from build123d import *

# Parameters (mm, degrees)
BOSS_EXTRUDE1_DEPTH = 88.9
FILLET1_R           = 10.16
CUT_EXTRUDE1_REACH  = 76.71
SKETCH2_R           = 3.429
SKETCH2_R_2         = 2.54
SKETCH2_W           = 45.212
SKETCH2_H           = 26.416
CUT_EXTRUDE3_REACH  = 83.026
SKETCH4_R           = 1.27
SKETCH4_W           = 27.94
SKETCH4_H           = 25.4


with BuildPart() as part:
    # Sketch1 → Boss-Extrude1 (new body)
    with BuildSketch(Plane(origin=(0, 0, 0), x_dir=(0, 0, -1), z_dir=(1, 0, 0))):
        Polygon((0, 0), (0, 23.315129188), (30.532870812, 53.848), (74.676, 53.848), (74.676, 0), (77.851, 0), (77.851, 57.023), (29.217742751, 57.023), (-3.175, 24.630257249), (-3.175, 0), align=None)
    extrude(amount=BOSS_EXTRUDE1_DEPTH)

    # Fillet1
    fillet1_edges = [part.edges().sort_by_distance(p)[0] for p in [
        (44.45, 24.630257249, 3.175),
        (44.45, 57.023, -29.217742751),
        (44.45, 57.023, -77.851),
        (44.45, 53.848, -74.676),
        (44.45, 53.848, -30.532870812),
        (44.45, 23.315129188, 0),
    ]]
    fillet(fillet1_edges, radius=FILLET1_R)

    # Sketch2 → Cut-Extrude1 (cut, up to next)
    with BuildSketch(Plane(origin=(0, 13.902628624, 13.902628624), x_dir=(1, 0, 0), z_dir=(0, 0.707106781, 0.707106781)), mode=Mode.PRIVATE) as cut_extrude1_sk1:
        with Locations(Location((75.819, 46.966285953, 0), (0, 0, 270))):  # turned: the seam where the file's is
            Circle(SKETCH2_R)
    cut_extrude1_tool1 = extrude(cut_extrude1_sk1.sketch, amount=-CUT_EXTRUDE1_REACH, mode=Mode.PRIVATE) & part.part
    add(cut_extrude1_tool1.solids().sort_by_distance((75.819, 47.112808, -19.307551))[0], mode=Mode.SUBTRACT)
    # Sketch2 → Cut-Extrude1 (cut, up to next)
    with BuildSketch(Plane(origin=(0, 13.902628624, 13.902628624), x_dir=(1, 0, 0), z_dir=(0, 0.707106781, 0.707106781)), mode=Mode.PRIVATE) as cut_extrude1_sk2:
        with Locations(Location((75.819, 29.186285953, 0), (0, 0, 270))):  # turned: the seam where the file's is
            Circle(SKETCH2_R)
    cut_extrude1_tool2 = extrude(cut_extrude1_sk2.sketch, amount=-CUT_EXTRUDE1_REACH, mode=Mode.PRIVATE) & part.part
    add(cut_extrude1_tool2.solids().sort_by_distance((75.819, 34.540449, -6.735192))[0], mode=Mode.SUBTRACT)
    # Sketch2 → Cut-Extrude1 (cut, up to next)
    with BuildSketch(Plane(origin=(0, 13.902628624, 13.902628624), x_dir=(1, 0, 0), z_dir=(0, 0.707106781, 0.707106781)), mode=Mode.PRIVATE) as cut_extrude1_sk3:
        with Locations(Location((59.436, 47.601285953, 0), (0, 0, 270))):  # turned: the seam where the file's is
            Circle(SKETCH2_R_2)
    cut_extrude1_tool3 = extrude(cut_extrude1_sk3.sketch, amount=-CUT_EXTRUDE1_REACH, mode=Mode.PRIVATE) & part.part
    add(cut_extrude1_tool3.solids().sort_by_distance((59.436, 47.561821, -19.756563))[0], mode=Mode.SUBTRACT)
    # Sketch2 → Cut-Extrude1 (cut, up to next)
    with BuildSketch(Plane(origin=(0, 13.902628624, 13.902628624), x_dir=(1, 0, 0), z_dir=(0, 0.707106781, 0.707106781)), mode=Mode.PRIVATE) as cut_extrude1_sk4:
        with Locations(Location((59.436, 28.551285953, 0), (0, 0, 270))):  # turned: the seam where the file's is
            Circle(SKETCH2_R_2)
    cut_extrude1_tool4 = extrude(cut_extrude1_sk4.sketch, amount=-CUT_EXTRUDE1_REACH, mode=Mode.PRIVATE) & part.part
    add(cut_extrude1_tool4.solids().sort_by_distance((59.436, 34.091437, -6.286179))[0], mode=Mode.SUBTRACT)
    # Sketch2 → Cut-Extrude1 (cut, up to next)
    with BuildSketch(Plane(origin=(0, 13.902628624, 13.902628624), x_dir=(1, 0, 0), z_dir=(0, 0.707106781, 0.707106781)), mode=Mode.PRIVATE) as cut_extrude1_sk5:
        with Locations((25.781, 38.076285953)):
            Rectangle(SKETCH2_W, SKETCH2_H)
    cut_extrude1_tool5 = extrude(cut_extrude1_sk5.sketch, amount=-CUT_EXTRUDE1_REACH, mode=Mode.PRIVATE) & part.part
    add(cut_extrude1_tool5.solids().sort_by_distance((25.781, 40.826629, -13.021371))[0], mode=Mode.SUBTRACT)

    # Sketch4 → Cut-Extrude3 (cut, up to next)
    with BuildSketch(Plane(origin=(0, 0, -77.851), x_dir=(-1, 0, 0), z_dir=(0, 0, -1)), mode=Mode.PRIVATE) as cut_extrude3_sk1:
        with Locations((-44.45, 3.81)):
            Circle(SKETCH4_R)
    cut_extrude3_tool1 = extrude(cut_extrude3_sk1.sketch, amount=-CUT_EXTRUDE3_REACH, mode=Mode.PRIVATE) & part.part
    add(cut_extrude3_tool1.solids().sort_by_distance((44.45, 3.81, -77.851))[0], mode=Mode.SUBTRACT)
    # Sketch4 → Cut-Extrude3 (cut, up to next)
    with BuildSketch(Plane(origin=(0, 0, -77.851), x_dir=(-1, 0, 0), z_dir=(0, 0, -1)), mode=Mode.PRIVATE) as cut_extrude3_sk2:
        with Locations((-17.145, 30.988)):
            Rectangle(SKETCH4_W, SKETCH4_H)
    cut_extrude3_tool2 = extrude(cut_extrude3_sk2.sketch, amount=-CUT_EXTRUDE3_REACH, mode=Mode.PRIVATE) & part.part
    add(cut_extrude3_tool2.solids().sort_by_distance((17.145, 30.988, -77.851))[0], mode=Mode.SUBTRACT)


solid = part.part
For this review, take the finished solid that the model builds, in its own axes (mm). A direction names the side the tool comes from. Give positions to 0.01 mm unless a question says otherwise; leave off trailing zeros. Write each loop counter-clockwise with the first axis right and the second up, starting at its lowest first coordinate (ties: lowest second). Pieces come first, ordered by that corner, then holes. Notation, with made-up numbers: (37, 39) -> (77, 39) arc R24 cw to (77, 52) -> close; hole circle Ø1 at (66.25, 69.5). An arc over 180 degrees is marked (long way). Use CSV: the item, a comma, the result in double quotes.
Q1. For P1, Ø1, axis at x = 13, z = -76, coming from the -Y side; P2, Ø12, axis at x = 50, y = 40.5, coming from the +Z side; P3, Ø5, axis at x = 40.5, y = 27.5, coming from the +Z side; P4, Ø1.5, axis at x = 52.5, z = -8.5, coming from the -Y side, all flat-tipped, find the tip position at first contact; note any pin that passes through.
Conclusion:
P1,"y = 0"
P2,"z = -6.69"
P3,"z = 2.09"
P4,"y = 31.07"
Q2. Take a section at C-C, the plane y = 14. Write out the cut boundary in (x, z) (3 decimals).
Conclusion:
outline,"(0, -77.851) -> (88.9, -77.851) -> (88.9, -74.676) -> (0, -74.676) -> close; (0, 0) -> (88.9, 0) -> (88.9, 3.175) -> (0, 3.175) -> close"
Q3. Mouldability with a two-part tool opening along Y and no side actions: class faces 6 (the face through (61.58, 45.49, -19.9)), 7 (the face through (44, 10, 3.175)), 8 (the face through (44, 0, -76)), 9 (the face through (25.46, 30.38, -4.79)) as pulls with the +Y half, pulls with the -Y half, needs draft (parallel to the pull), parting line crosses it, or undercut.
Conclusion:
face 6,"undercut"
face 7,"needs draft"
face 8,"pulls with the -Y half"
face 9,"pulls with the +Y half"
Q4. Take a section at B-B, the plane x = 44.45. Write out the cut boundary in (y, z) (3 decimals).
Conclusion:
outline,"(0, -77.851) -> (2.54, -77.851) -> (2.54, -74.676) -> (0, -74.676) -> close; (0, 0) -> (19.107, 0) arc R10.16 cw to (26.291, -2.976) -> (29.242, -5.927) -> (31.487, -3.682) -> (27.606, 0.199) arc R10.16 ccw to (20.422, 3.175) -> (0, 3.175) -> close; (5.08, -77.851) -> (46.863, -77.851) arc R10.16 ccw to (57.023, -67.691) -> (57.023, -33.426) arc R10.16 ccw to (54.047, -26.242) -> (50.166, -22.361) -> (47.921, -24.606) -> (50.872, -27.557) arc R10.16 cw to (53.848, -34.741) -> (53.848, -64.516) arc R10.16 cw to (43.688, -74.676) -> (5.08, -74.676) -> close"
Q5. Take a section at D-D, the plane x = 23.5. Write out the cut boundary in (y, z) (3 decimals), then the cut area to 3 significant figures.
Conclusion:
outline,"(0, -77.851) -> (18.288, -77.851) -> (18.288, -74.676) -> (0, -74.676) -> close; (0, 0) -> (19.107, 0) arc R10.16 cw to (26.291, -2.976) -> (29.242, -5.927) -> (31.487, -3.682) -> (27.606, 0.199) arc R10.16 ccw to (20.422, 3.175) -> (0, 3.175) -> close; (43.688, -77.851) -> (46.863, -77.851) arc R10.16 ccw to (57.023, -67.691) -> (57.023, -33.426) arc R10.16 ccw to (54.047, -26.242) -> (50.166, -22.361) -> (47.921, -24.606) -> (50.872, -27.557) arc R10.16 cw to (53.848, -34.741) -> (53.848, -64.516) arc R10.16 cw to (43.688, -74.676) -> close"
area,"376 mm2"
Q6. Tool access review of faces 1 (the face through (25.465, 49.059, -23.468)), 2 (the face through (17, 43.688, -76)), 3 (the face through (31.115, 31, -76)), 4 (the face through (0, 54, -43)), 5 (the face through (45.072, 53.053, -30.802)): name each direction out of +Z, -Z, +X, -X, +Y, -Y from which nothing blocks a thin tool from reaching the whole face with its end or side.
Conclusion:
face 1,"+Z, -Y"
face 2,"+Z, -Z"
face 3,"-Z"
face 4,"+Z, -Z, -X, +Y, -Y"
face 5,"+X, -X, -Y"
Q7. Take a section at A-A, the plane y = 3.81. Write out the cut boundary in (x, z) (3 decimals), then the cut area to 3 significant figures.
Conclusion:
outline,"(0, -77.851) -> (43.18, -77.851) -> (43.18, -74.676) -> (0, -74.676) -> close; (0, 0) -> (88.9, 0) -> (88.9, 3.175) -> (0, 3.175) -> close; (45.72, -77.851) -> (88.9, -77.851) -> (88.9, -74.676) -> (45.72, -74.676) -> close"
area,"556 mm2"
Q8. To check wall thickness, follow probe 1 along Z at (x, y) = (62.5, 8.5) (3 decimals); probe 2 along Z at (x, y) = (39.5, 52.5); probe 3 along Y at (x, z) = (44, -75). State the ranges of each line that lie inside material, in increasing order. Write a range as [from, to].
Conclusion:
probe 1,"[-77.851, -74.676], [0, 3.175]"
probe 2,"[-76.14, -69.57], [-29.68, -24.69]"
probe 3,"[0, 2.62], [5, 53.92]"
